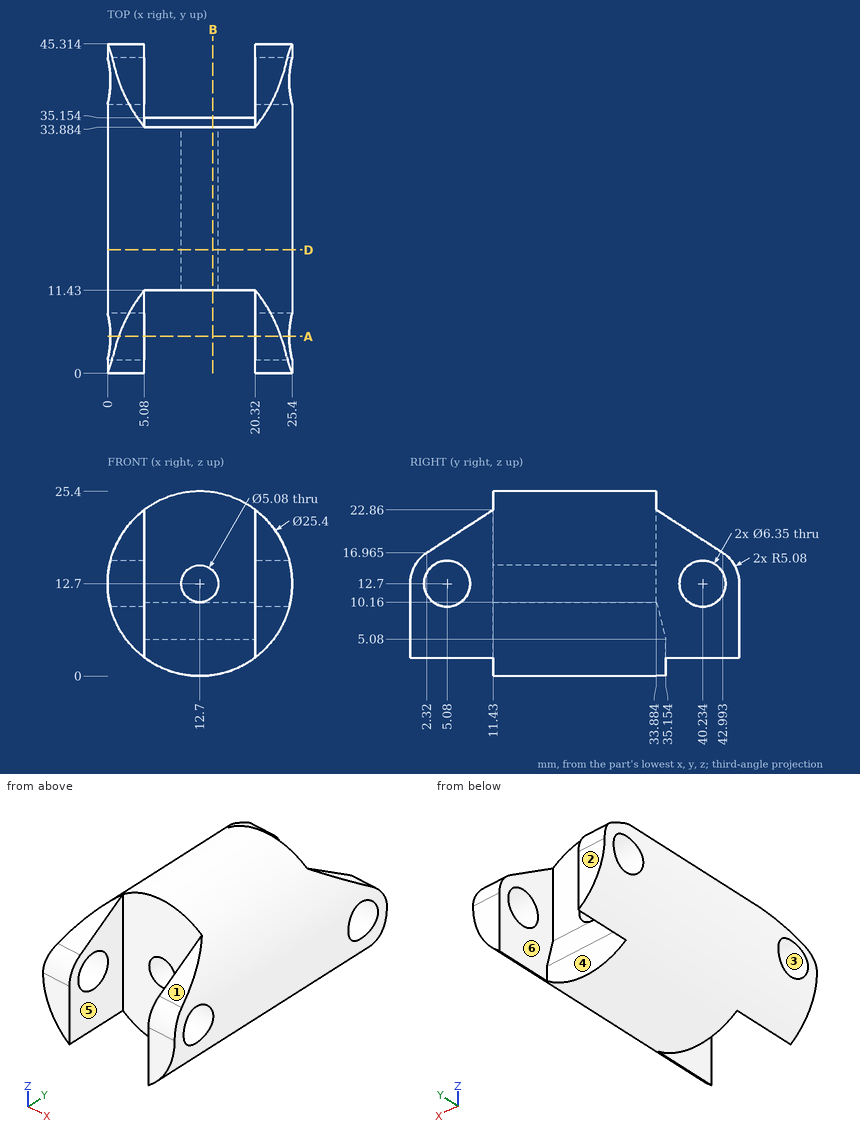
Drawing for the job (mm, zero at the part's lowest x, y, z). A direction names the side the tool comes from. Coordinates: 2 decimals unless noted, no trailing zeros. Loops run counter-clockwise (first coordinate to the right, second up) from the corner with the lowest first, then second, coordinate; pieces in that order, holes last. Notation, with made-up numbers: (10, 15.25) - (18, 15.25) arc R23 ccw to (18, 48.25) - close; hole circle Ø4 at (71.25, 23.5). An arc over 180 degrees is marked (long way). Return JSON: item names as keys, results as strings.
1. Band-saw the part on B-B (x = 14.5). Give the cut face in (y, z).
Result:
{"outline": "(11.43, 0.13) - (35.15, 0.13) - (35.15, 5.08) - (33.88, 10.16) - (33.88, 10.91) - (11.43, 10.91) - close; (11.43, 14.49) - (33.88, 14.49) - (33.88, 25.27) - (11.43, 25.27) - close"}
2. Mould opens along Z. For the marked faces 1, 2 and 3 say: released by +Z, released by -Z, zero draft, split by the parting line, or undercut.
Result:
{"face 1": "released by +Z", "face 2": "zero draft", "face 3": "undercut"}
3. Band-saw the part on D-D (y = 17). Give the cut face in (x, z).
Result:
{"outline": "circle Ø25.4 at (12.7, 12.7); hole circle Ø5.08 at (12.7, 12.7)"}
4. Drop flat-ended pins along their axis: pin 1 (5.5 mm diameter, centred on y = 40, z = 14.5, fed in from +X); pin 2 (10 mm diameter, centred on y = 6.5, z = 6.5, fed in from -X); pin 3 (8 mm diameter, centred on x = 21, y = 30, fed in from -Z); pin 4 (5.5 mm diameter, centred on y = 40.23, z = 12.7, fed in from -X). Give the stop position or say it passes through.
Result:
{"pin 1": "stops at x = 25.34", "pin 2": "stops at x = 0.08", "pin 3": "stops at z = 0.75", "pin 4": "passes through"}
5. Probe L1, parallel to X at y = 9, z = 13; L2, parallel to X at y = 35, z = 19.75 (1 decimal); L3, parallel to Y at x = 15.75, z = 16.5. List the from-to ranges inside material, lowest first. Write a range as from..to.
Result:
{"L1": "x = 0..5.08, 20.32..25.4", "L2": "x = 2.1..5.1, 20.3..23.3", "L3": "y = 11.43..33.88"}
6. Band-saw the part on A-A (y = 5.08). State how many separate pieces and enclosed holes the cut face has.
Result:
{"separate pieces": "4", "enclosed holes": "0"}
7. 3-axis set-ups, long thin cutter, end or side, ignore diameter. For the marked faces 4, 5 and 6: which of +Z, -Z, +X, -X, +Y, -Y reach the whole face in a straight line?
Result:
{"face 4": "+Z, -Z, +Y", "face 5": "+Z, -Z, -Y", "face 6": "+Z, +Y"}
